Check sheet for the modelled part. Datum: model origin and axes. Units: mm. A direction names the side the tool comes from. Coordinates: 2 decimals unless noted, no trailing zeros. Loops run counter-clockwise (first coordinate to the right, second up) from the corner with the lowest first, then second, coordinate; pieces in that order, holes last. Notation, with made-up numbers: M 67.5,72.5 L 117.5,72.5 A21 ccw 117.5,92.5 Z; hole C 66.25,80 d10. An arc over 180 degrees is marked long. Use CSV: the item, a comma, the result in double quotes. Start each with the question number.
(1) Section check D-D on x = 5. Record the cut outline in (y, z).
(2) Section check A-A on x = 1.75. Record the cut outline in (y, z).
(3) Section check B-B on z = 18.5. Record the cut outline in (x, y).
(4) Draft check along X on faces 6 (the cylindrical face through (7.243, 3.479, 16.972)), 7 (the flat face through (1, 30.5, 15)), 8 (the flat face through (6.2, 26, 15)). Enter one of: pulls with the +X half, pulls with the -X half, needs draft (parallel to the pull), parting line crosses it, or undercut.
(5) Scan lines: line 1 (Y direction, x = 4, z = 18.05); line 2 (Z direction, x = 4.25, y = 26.5); line 3 (Y direction, x = 5, z = 14.25). Record each from-to range of solid material in increasing order.
(6) Go/stop test with flat-tipped pins: pin 1 Ø3 at (x, z) = (3, 22.5) entering from -Y; pin 2 Ø1.5 at (x, z) = (1, 19.5) entering from -Y; pin 3 Ø1.1 at (x, z) = (1.5, 6) entering from -Y. Record where each tip stops, or that it passes through.
(7) Set-up check for faces 1 (the flat face through (2, 8, 19)), 2 (the flat face through (3, 8, 15)), 3 (the flat face through (1, 24, 0)), 4 (the flat face through (-0.5, 16, 15)), 5 (the flat face through (1, 27, 30)): record each of +Z, -Z, +X, -X, +Y, -Y from which the full face is reachable in a straight line by a thin tool's end or side.
(8) Section check C-C on z = 27.75. Record the cut outline in (x, y).
from build123d import *

# Parameters (mm, degrees)
F1_DEPTH     = 19
F3_DEPTH     = 11
F4_R         = 3.4
F5_DEPTH     = 25
F8_DEPTH     = 25
F9_T1_DEPTH  = 55.1336597593
F10_DEPTH    = 15
F11_T1_DEPTH = 3.7
F11_T3_DEPTH = 12.9815131525


# Not quite as in the source:
# - a fillet or chamfer that OpenCascade refuses, or shapes differently, is made with other operations: its cross-section is extruded or revolved along the edge and cut away or added


with BuildPart() as f1:
    # F0 (on Top) → F1 (new body)
    with BuildSketch(Plane.XY):
        with BuildLine():
            ThreePointArc((4, 0), (7.1819805153, 1.3180194847), (8.5, 4.5))
            ThreePointArc((8.5, 4.5), (6.8853076093, 7.95325933), (3.2, 8.9283179651))
            ThreePointArc((3.2, 8.9283179651), (0.54674067, 7.3853076093), (-0.5, 4.5))
            ThreePointArc((-0.5, 4.5), (0.8180194847, 1.3180194847), (4, 0))
        make_face()
        with BuildLine():
            ThreePointArc((-0.5, 4.5), (0.54674067, 7.3853076093), (3.2, 8.9283179651))
            Line((3.2, 8.9283179651), (3.2, 22.5))
            Line((3.2, 22.5), (6.2, 22.5))
            Line((6.2, 22.5), (6.2, 30.5))
            Line((6.2, 30.5), (-3.5, 30.5))
            Line((-3.5, 30.5), (-3.5, 22.5))
            Line((-3.5, 22.5), (-0.5, 22.5))
            Line((-0.5, 22.5), (-0.5, 4.5))
        make_face()
    extrude(amount=F1_DEPTH)

    # F2 (on face) → F3 (join)
    with BuildSketch(Plane.XY.offset(19)):
        Polygon((6.2, 30.5), (-3.5, 30.5), (-3.5, 22.5), (-0.5, 22.5), (-0.5, 12.5), (3.2, 12.5), (3.2, 22.5), (6.2, 22.5), align=None)
    extrude(amount=F3_DEPTH)

    # F4 (on face) → F5 (cut)
    with BuildSketch(Plane(origin=(0, 0, 0), x_dir=(1, 0, 0), z_dir=(0, 0, -1))):
        with Locations((4, -4.5)):
            Circle(F4_R)
    extrude(amount=-F5_DEPTH, mode=Mode.SUBTRACT)

    # F7 (on face) → F8 (cut)
    with BuildSketch(Plane(origin=(-3.5, 0, 0), x_dir=(0, -1, 0), z_dir=(-1, 0, 0))):
        with BuildLine():
            ThreePointArc((-26.5, 7.5), (-25.4393398282, 7.9393398282), (-25, 9))
            ThreePointArc((-25, 9), (-27.5606601718, 10.0606601718), (-26.5, 7.5))
        make_face()
    extrude(amount=-F8_DEPTH, mode=Mode.SUBTRACT)

    # F9: chamfer of 10 on 1 edges, made by hand

    # F9_s2 → F9_t1 (cut)
    with BuildSketch(Plane.YZ.offset(-26.2168298797)):
        Polygon((12.5, 20), (22.5, 30), (12.5, 30), align=None)
    extrude(amount=F9_T1_DEPTH, mode=Mode.SUBTRACT)

    # F6 (on Top) → F10 (cut)
    with BuildSketch(Plane.XY):
        Polygon((-2.952047158, 0), (0, 0), (4.1492179482, 0), (5.4492179482, 0), (9.2530830997, 0), (9.2530830997, 9.0487509014), (9.2530830997, 14.2418248579), (-2.952047158, 14.2418248579), align=None)
    extrude(amount=F10_DEPTH, mode=Mode.SUBTRACT)

    # F11: fillet of radius 5 on 2 edges, made by hand

    # F11_s2 → F11_t1 (join)
    with BuildSketch(Plane.YZ.offset(-0.5)):
        with BuildLine():
            ThreePointArc((14.2418248579, 10), (12.7773587638, 13.5355339059), (9.2418248579, 15))
            Line((9.2418248579, 15), (14.2418248579, 15))
            Line((14.2418248579, 15), (14.2418248579, 10))
        make_face()
    extrude(amount=F11_T1_DEPTH)

    # F11_s4 → F11_t3 (cut)
    with BuildSketch(Plane.YZ.offset(-5.1407565762)):
        with BuildLine():
            ThreePointArc((13.812604178, 21.312604178), (12.9997448715, 20.2451619378), (12.5, 19))
            Line((12.5, 19), (12.5, 20))
            Line((12.5, 20), (13.812604178, 21.312604178))
        make_face()
    extrude(amount=F11_T3_DEPTH, mode=Mode.SUBTRACT)


solid = f1.part
Outcome:
1,outline,"M 0.11,15 L 1.25,15 L 1.25,19 L 0.11,19 Z; M 7.75,15 L 8.89,15 L 8.89,19 L 7.75,19 Z; M 22.5,0 L 30.5,0 L 30.5,30 L 22.5,30 Z; hole C 26.5,9 d3"
2,outline,"M 0.6,15 L 1.95,15 L 1.95,19 L 0.6,19 Z; M 7.05,15 L 9.24,15 A5 cw 14.24,10 L 14.24,0 L 30.5,0 L 30.5,30 L 22.5,30 L 13.81,21.31 A5 ccw 12.5,19 L 7.05,19 Z; hole C 26.5,9 d3"
3,outline,"M -3.5,22.5 L -0.5,22.5 L -0.5,4.5 A4.5 ccw long 3.2,8.93 L 3.2,22.5 L 6.2,22.5 L 6.2,30.5 L -3.5,30.5 Z; hole C 4,4.5 d6.8"
4,face 6,"undercut"
4,face 7,"needs draft"
4,face 8,"pulls with the +X half"
5,line 1,"y = 0 to 1.1, 7.9 to 9, 22.5 to 30.5"
5,line 2,"z = 0 to 7.5, 10.5 to 30"
5,line 3,"y = 22.5 to 30.5"
6,pin 1,"stops at y = 13.53"
6,pin 2,"stops at y = 0.72"
6,pin 3,"stops at y = 14.24"
7,face 1,"+Z, +X, -X, -Y"
7,face 2,"-Z, +X, -X, -Y"
7,face 3,"-Z, +X, -X, +Y, -Y"
7,face 4,"+Z, -Z, -X, -Y"
7,face 5,"+Z, +X, -X, +Y, -Y"
8,outline,"M -3.5,22.5 L -0.5,22.5 L -0.5,20.25 L 3.2,20.25 L 3.2,22.5 L 6.2,22.5 L 6.2,30.5 L -3.5,30.5 Z"
